Source: CAD feature listing. Evaluate the final solid. Frame: model axes, mm. A direction names the side the tool comes from. Round coordinates to 2 decimals unless told otherwise and drop trailing zeros. Loops run counter-clockwise (first coordinate to the right, second up) from the corner with the lowest first, then second, coordinate; pieces in that order, holes last. Notation, with made-up numbers: M -36,9.5 L -7,9.5 A16 cw -7,20.5 Z; hole C -27.5,-32.75 d7. An arc over 180 degrees is marked long. One line per item, written item: value.
from build123d import *

# Parameters (mm, degrees)
SKETCH1_R           = 5.4
BOSS_EXTRUDE1_DEPTH = 25.75
SKETCH2_W           = 2.5
SKETCH2_H           = 5.463227165
BOSS_EXTRUDE2_DEPTH = 5
FILLET1_R           = 1
FILLET2_R           = 0.25
SKETCH4_R           = 2.875
CUT_EXTRUDE1_DEPTH  = 25.75
SKETCH5_R           = 4.375
CUT_EXTRUDE2_DEPTH  = 0.9
SKETCH6_R           = 4.375
CUT_EXTRUDE3_DEPTH  = 0.9
SKETCH9_W           = 2.6
SKETCH9_H           = 6.5
CUT_EXTRUDE4_DEPTH  = 10


with BuildPart() as part:
    # Sketch1 → Boss-Extrude1 (new body)
    with BuildSketch(Plane(origin=(0, 0, 0), x_dir=(1, 0, 0), z_dir=(0, 1, 0))):
        Circle(SKETCH1_R)
    extrude(amount=BOSS_EXTRUDE1_DEPTH)

    # Sketch2 → Boss-Extrude2 (add)
    with BuildSketch(Plane.XZ):
        Polygon((2.738101985, -0.137468245), (7.46660069, -2.867468245), (6.21660069, -5.032531755), (1.488101985, -2.302531755), align=None)
        with Locations((0, 5.168386418)):
            Rectangle(SKETCH2_W, SKETCH2_H)
        Polygon((-2.738101985, -0.137468245), (-1.488101985, -2.302531755), (-6.21660069, -5.032531755), (-7.46660069, -2.867468245), align=None)
    extrude(amount=-BOSS_EXTRUDE2_DEPTH)

    # Fillet1
    fillet1_edges = [part.edges().sort_by_distance(p)[0] for p in [
        (0, 5, 7.9),
        (0, 0, 7.9),
        (6.84160069, 5, -3.95),
        (6.84160069, 0, -3.95),
        (-6.84160069, 5, -3.95),
        (-6.84160069, 0, -3.95),
    ]]
    fillet(fillet1_edges, radius=FILLET1_R)

    # Fillet2
    fillet2_edges = [part.edges().sort_by_distance(p)[0] for p in [
        (-5.4, 25.75, 0),
    ]]
    fillet(fillet2_edges, radius=FILLET2_R)

    # Sketch4 → Cut-Extrude1 (cut)
    with BuildSketch(Plane.XZ):
        Circle(SKETCH4_R)
    extrude(amount=-CUT_EXTRUDE1_DEPTH, mode=Mode.SUBTRACT)

    # Sketch5 → Cut-Extrude2 (cut)
    with BuildSketch(Plane(origin=(0, 0, 0), x_dir=(-1, 0, 0), z_dir=(0, -1, 0))):
        Circle(SKETCH5_R)
    extrude(amount=-CUT_EXTRUDE2_DEPTH, mode=Mode.SUBTRACT)

    # Sketch6 → Cut-Extrude3 (cut)
    with BuildSketch(Plane(origin=(0, 25.75, 0), x_dir=(1, 0, 0), z_dir=(0, 1, 0))):
        Circle(SKETCH6_R)
    extrude(amount=-CUT_EXTRUDE3_DEPTH, mode=Mode.SUBTRACT)

    # Sketch9 → Cut-Extrude4 (cut)
    with BuildSketch(Plane(origin=(0, 0, 0), x_dir=(0.866025404, 0, 0.5), z_dir=(-0.5, 0, 0.866025404))):
        with Locations((0.244134383, 7.25)):
            Rectangle(SKETCH9_W, SKETCH9_H)
    extrude(amount=CUT_EXTRUDE4_DEPTH, mode=Mode.SUBTRACT)


solid = part.part
1. Section query B-B (y = 17.75). Return the cut outline in (x, z) (3 decimals), and give its area (3 significant figures).
Report:
outline: C 0,0 d10.8; hole C 0,0 d5.75
area: 65.6 mm2
2. Ray query, line 1 (Z direction, x = 0, y = 15.75) (3 decimals); line 2 (Y direction, x = 1, z = 5.5); line 3 (X direction, y = 12, z = -1.25). Return the intervals inside material, ascending. Write a range as [from, to].
Report:
line 1: z = [-5.4, -2.875], [2.875, 5.4]
line 2: y = [0, 5]
line 3: x = [-5.25, -2.59], [2.59, 5.25]
3. Reachability of faces 4 (the face through (5, 5, -3)), 5 (the face through (3.472, 0.444, 2.662)), 6 (the face through (-5, 5, -3)) from +Z, -Z, +X, -X, +Y, -Y: full face, straight path, thin tool, end or side. Return the list, or none.
Report:
face 4: -Z, +X, +Y
face 5: -Y
face 6: -Z, -X, +Y
4. Pull-direction query (Z, two-part tool) for faces 1 (the face through (-1.25, 2, 7)), 2 (the face through (-6.83, 2.48, -3.97)), 3 (the face through (-0.553, 7.204, 4.046)); classes: released by +Z, released by -Z, zero draft, split by the parting line, or undercut.
Report:
face 1: zero draft
face 2: released by -Z
face 3: undercut
5. Section query A-A (z = 0). Return the cut outline in (x, y) (3 decimals).
Report:
outline: M -5.4,0 L -4.375,0 L -4.375,0.9 L -2.875,0.9 L -2.875,24.85 L -4.375,24.85 L -4.375,25.75 L -5.15,25.75 A0.25 ccw -5.4,25.5 Z; M 2.875,0.9 L 4.375,0.9 L 4.375,0 L 5.4,0 L 5.4,25.5 A0.25 ccw 5.15,25.75 L 4.375,25.75 L 4.375,24.85 L 2.875,24.85 Z
6. Pin query (flat end, axial travel): pin 1 (4 mm diameter, centred on y = 20, z = -3.5, fed in from -X); pin 2 (0.8 mm diameter, centred on x = 6, z = -3, fed in from +Y); pin 3 (4 mm diameter, centred on y = 10, z = 3, fed in from +X); pin 4 (5 mm diameter, centred on x = 0, z = 0, fed in from -Y). Return the tip coordinate at first contact, or that it passes through.
Report:
pin 1: stops at x = -5.19
pin 2: stops at y = 5
pin 3: stops at x = 5.31
pin 4: passes through
7. Section query C-C (y = 4.5). Return the cut outline in (x, z) (3 decimals), and give its area (3 significant figures).
Report:
outline: M -7.351,-2.8 L -6.101,-4.966 L -3.925,-3.709 A5.4 ccw 3.925,-3.709 L 6.101,-4.966 L 7.351,-2.8 L 5.175,-1.544 A5.4 ccw 1.25,5.253 L 1.25,7.766 L -1.25,7.766 L -1.25,5.253 L 0.125,2.872 A2.875 cw long -2.251,1.788 L -3.562,4.058 A5.4 ccw -5.175,-1.544 Z
area: 77.0 mm2
8. Section query D-D (y = 9.75). Return the cut outline in (x, z) (3 decimals).
Report:
outline: M -3.562,4.058 A5.4 ccw long -1.25,5.253 L 0.125,2.872 A2.875 cw long -2.251,1.788 Z
